Work out the finished part from the listing and answer in its coordinate system (mm). A direction names the side the tool comes from. Coordinates: 2 decimals unless noted, no trailing zeros. Loops run counter-clockwise (first coordinate to the right, second up) from the corner with the lowest first, then second, coordinate; pieces in that order, holes last. Notation, with made-up numbers: (89, 21) -> (109, 21) arc R17 cw to (109, 51) -> close; hole circle Ø3 at (79.25, -4). An arc over 180 degrees is marked (long way). One line per question, with ' | ' between items.
```python
from build123d import *

# Parameters (mm, degrees)
SKETCH1_W           = 3.8354
SKETCH1_H           = 15
BOSS_EXTRUDE1_DEPTH = 2.667
SKETCH4_R           = 0.8
CUT_EXTRUDE1_DEPTH  = 1.9177
SKETCH5_R           = 0.64
CUT_EXTRUDE2_DEPTH  = 2.9177
SKETCH6_R           = 0.69
CUT_EXTRUDE3_DEPTH  = 1.27
SKETCH9_W           = 3.8354
SKETCH9_H           = 2.667
CUT_EXTRUDE5_DEPTH  = 1.2


with BuildPart() as part:
    # Sketch1 → Boss-Extrude1 (new body)
    with BuildSketch(Plane(origin=(0, 0, 0), x_dir=(1, 0, 0), z_dir=(0, 1, 0))):
        Rectangle(SKETCH1_W, SKETCH1_H)
    extrude(amount=BOSS_EXTRUDE1_DEPTH)

    # Sketch4 → Cut-Extrude1 (cut)
    with BuildSketch(Plane(origin=(1.9177, 0, 0), x_dir=(0, 0, -1), z_dir=(1, 0, 0))):
        with Locations((-6.328069737, 1.3335)):
            Circle(SKETCH4_R)
        with Locations((-4.423069737, 1.3335)):
            Circle(SKETCH4_R)
        with Locations((-2.518069737, 1.3335)):
            Circle(SKETCH4_R)
        with Locations((-0.613069737, 1.3335)):
            Circle(SKETCH4_R)
        with Locations((1.291930263, 1.3335)):
            Circle(SKETCH4_R)
        with Locations((3.196930263, 1.3335)):
            Circle(SKETCH4_R)
        with Locations((5.101930263, 1.3335)):
            Circle(SKETCH4_R)
    extrude(amount=-CUT_EXTRUDE1_DEPTH, mode=Mode.SUBTRACT)

    # Sketch5 → Cut-Extrude2 (cut, through all)
    with BuildSketch(Plane(origin=(0, 0, 0), x_dir=(0, 0, -1), z_dir=(1, 0, 0))):
        with Locations((-6.328069737, 1.3335)):
            Circle(SKETCH5_R)
        with Locations((-4.423069737, 1.3335)):
            Circle(SKETCH5_R)
        with Locations((-2.518069737, 1.3335)):
            Circle(SKETCH5_R)
        with Locations((-0.613069737, 1.3335)):
            Circle(SKETCH5_R)
        with Locations((1.291930263, 1.3335)):
            Circle(SKETCH5_R)
        with Locations((3.196930263, 1.3335)):
            Circle(SKETCH5_R)
    extrude(amount=-CUT_EXTRUDE2_DEPTH, mode=Mode.SUBTRACT)

    # Sketch6 → Cut-Extrude3 (cut)
    with BuildSketch(Plane(origin=(0, 0, 0), x_dir=(0, 0, -1), z_dir=(1, 0, 0))):
        with Locations((5.101930263, 1.3335)):
            Circle(SKETCH6_R)
    extrude(amount=-CUT_EXTRUDE3_DEPTH, mode=Mode.SUBTRACT)

    # Sketch9 → Cut-Extrude5 (cut)
    with BuildSketch(Plane(origin=(0, 0, -7.5), x_dir=(-1, 0, 0), z_dir=(0, 0, -1))):
        with Locations((0, 1.3335)):
            Rectangle(SKETCH9_W, SKETCH9_H)
    extrude(amount=-CUT_EXTRUDE5_DEPTH, mode=Mode.SUBTRACT)


solid = part.part
```
1) Flat-ended cylindrical pins translate along their axes: pin 1 (0.7 mm diameter, centred on y = 1.5, z = -5, fed in from +X); pin 2 (1.3 mm diameter, centred on y = 1.5, z = -1, fed in from +X); pin 3 (1.5 mm diameter, centred on y = 1.33, z = -3.2, fed in from +X). Find the tip coordinate at first contact, or state that the pin passes through.
Check values:
pin 1: stops at x = -1.27 | pin 2: stops at x = 1.92 | pin 3: stops at x = 0
2) The mould has two halves that part along Z. Classify faces 1 (the face through (0, 2.667, 1)), 2 (the face through (0, 1, -6.3)), 3 (the face through (-0.95, 1.09, 3.83)): released by +Z, released by -Z, zero draft, split by the parting line, or undercut.
Check values:
face 1: zero draft | face 2: released by -Z | face 3: undercut
3) Find the intervals of material crossed by line 1 along Y through (x, z) = (-1.75, 6.25); line 2 along Y through (x, z) = (1.1, 5.75); line 3 along X through (y, z) = (1.75, -3.75), in increasing order.
Check values:
line 1: y = 0 to 0.7, 1.97 to 2.67 | line 2: y = 0 to 0.78, 1.89 to 2.67 | line 3: x = -1.92 to 0
4) Find section B-B (x = -1.05). Write down the section's boundary in (y, z), plus the area to 3 significant figures.
Check values:
outline: (0, -6.3) -> (2.67, -6.3) -> (2.67, 7.5) -> (0, 7.5) -> close; hole circle Ø1.38 at (1.33, -5.1); hole circle Ø1.28 at (1.33, -3.2); hole circle Ø1.28 at (1.33, -1.29); hole circle Ø1.28 at (1.33, 0.61); hole circle Ø1.28 at (1.33, 2.52); hole circle Ø1.28 at (1.33, 4.42); hole circle Ø1.28 at (1.33, 6.33) | area: 27.6 mm^2
5) Find section D-D (x = 0.85). Write down the section's boundary in (y, z).
Check values:
outline: (0, -6.3) -> (2.67, -6.3) -> (2.67, 7.5) -> (0, 7.5) -> close; hole circle Ø1.6 at (1.33, -5.1); hole circle Ø1.6 at (1.33, -3.2); hole circle Ø1.6 at (1.33, -1.29); hole circle Ø1.6 at (1.33, 0.61); hole circle Ø1.6 at (1.33, 2.52); hole circle Ø1.6 at (1.33, 4.42); hole circle Ø1.6 at (1.33, 6.33)
6) Find section A-A (z = 1). Write down the section's boundary in (x, y), plus the area to 3 significant figures.
Check values:
outline: (-1.92, 0) -> (1.92, 0) -> (1.92, 0.63) -> (0, 0.63) -> (0, 0.82) -> (-1.92, 0.82) -> close; (-1.92, 1.84) -> (0, 1.84) -> (0, 2.03) -> (1.92, 2.03) -> (1.92, 2.67) -> (-1.92, 2.67) -> close | area: 5.59 mm^2
7) Find section C-C (y = 1.05). State how many separate pieces and enclosed holes the cut face has, plus the area to 3 significant figures.
Check values:
separate pieces: 7 | enclosed holes: 0 | area: 18.0 mm^2
8) For faces 4 (the face through (1.918, 2.5, 0.7)), 5 (the face through (0.97, 1.03, -2.03)), determine the directions among +Z, -Z, +X, -X, +Y, -Y from which every point of the face is accessible in a straight line to the end or side of a thin tool.
Check values:
face 4: +Z, -Z, +X, +Y, -Y | face 5: +X
